For this review, use the dimensioned drawing (mm, ordinates from the lowest corner) and the shaded views. A direction names the side the tool comes from. Round coordinates to 2 decimals unless told otherwise and drop trailing zeros. Write each loop counter-clockwise with the first axis right and the second up, starting at its lowest first coordinate (ties: lowest second). Pieces come first, ordered by that corner, then holes. Notation, with made-up numbers: M 69.25,-26.75 L 124.25,-26.75 A37 cw 124.25,9.25 Z; hole C 2.25,87 d3. An arc over 180 degrees is marked long. Use one line per item in the form item = value. Start each with the question number.
Item 1: For line 1 (X direction, y = 24.75, z = 12.25), list the stretches that pass through material, from the lowest coordinate up. Write a range as [from, to].
Item 2: For P1, Ø0.5, axis at x = 16.5, y = 0.5, coming from the +Z side; P2, Ø7, axis at x = 15, z = 15, coming from the +Y side; P3, Ø6, axis at y = 22, z = 12, coming from the +X side; P4, Ø12, axis at x = 20.5, y = 25.5, coming from the +Z side, all flat-tipped, find the tip position at first contact; note any pin that passes through.
Item 3: For the marked faces 1 and 2, list the 3-axis set-ups (+Z, -Z, +X, -X, +Y, -Y) from which the entire face can be reached by the end or side of a thin tool; tool diameter is ignored.
Item 4: Add section A-A (x = 15). State the section outline as (y, z) points, and give its area (3 significant figures).
Item 5: Draft analysis for pull direction Y (two halves, no side actions). For the marked faces 3, 4, 5 and 6, state which applies: released by +Y, released by -Y, zero draft, split by the parting line, or undercut.
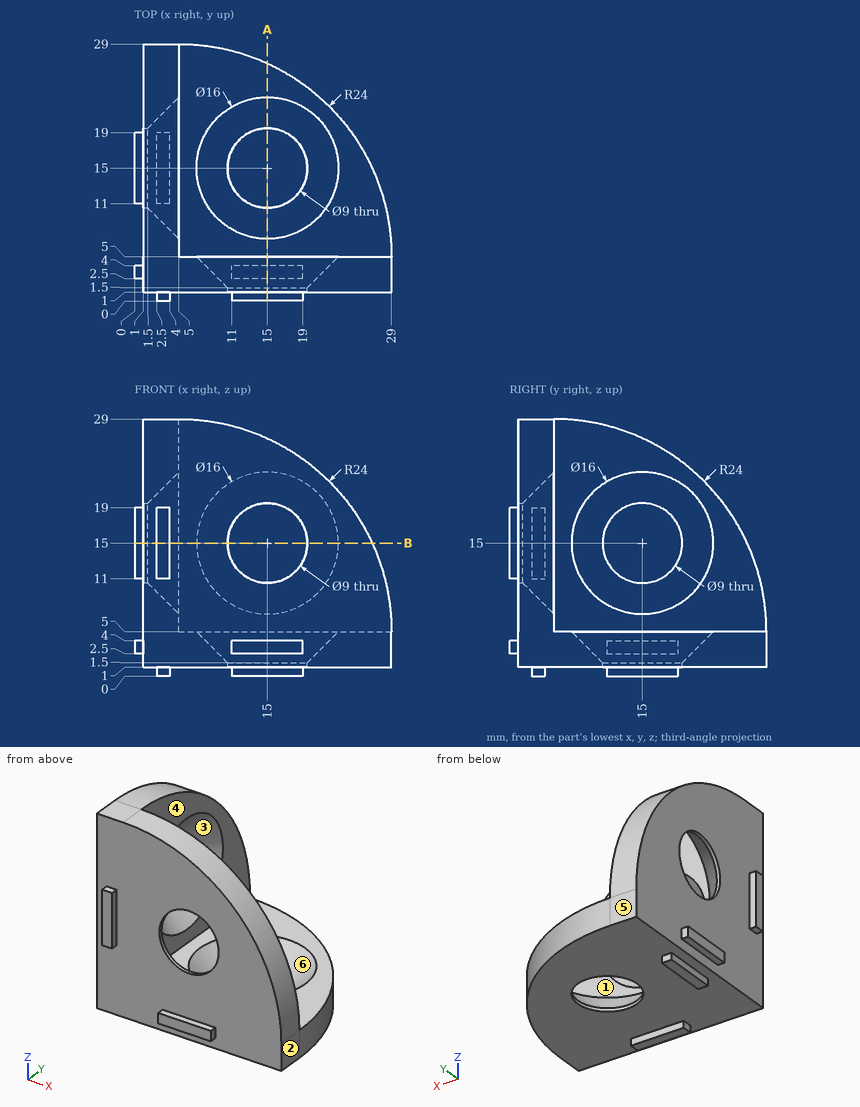
Calculated:
q1.line_1 = [1, 5]
q2.P1 = 4
q2.P2 = through
q2.P3 = 5
q2.P4 = 5
q3.face_1 = +Z, +X, +Y
q3.face_2 = +Z, -Z, +X, +Y, -Y
q4.outline = M 0,2.5 L 1,2.5 L 1,1 L 2.5,1 L 2.5,0 L 4,0 L 4,1 L 10.5,1 L 10.5,1.5 L 7,5 L 5,5 L 5,7 L 1.5,10.5 L 1,10.5 L 1,4 L 0,4 Z; M 1,19.5 L 1.5,19.5 L 5,23 L 5,26.82 L 1,26.82 Z; M 19.5,1 L 26.82,1 L 26.82,5 L 23,5 L 19.5,1.5 Z
q4.area = 97.0 mm^2
q5.face_3 = undercut
q5.face_4 = zero draft
q5.face_5 = released by +Y
q5.face_6 = undercut
